Source: CAD feature listing. Evaluate the final solid. Frame: model axes, mm. A direction names the side the tool comes from. Give positions to 0.01 mm unless a question says otherwise; leave off trailing zeros. Loops run counter-clockwise (first coordinate to the right, second up) from the corner with the lowest first, then second, coordinate; pieces in that order, holes last. Notation, with made-up numbers: (43.5, -32) -> (89.5, -32) arc R24 cw to (89.5, -12) -> close; hole circle Ø10 at (28, 80.25). An arc over 180 degrees is marked (long way). Return JSON: item names as keys, results as strings. Group by question number.
(1) Cut plane A-A on z = 18.5. Return loops of the section in (x, y).
(2) Cut plane C-C on x = 22. Return loops of the section in (y, z), then the cut area to 3 significant figures.
(3) Ray query, line 1 (X direction, y = 58, z = 26); line 2 (Z direction, x = 38, y = 26.5); line 3 (Y direction, x = 54, z = 23.5). Return the intervals inside material, ascending. Write a range as from..to.
(4) Access query for faces 1 (the face through (50, 42, 12.7)), 2 (the face through (0, 38, 26)). Directions: +Z, -Z, +X, -X, +Y, -Y. A direction counts if a zero-diameter tool reaches every point of the face in a straight line with its end or side. Return the directions, or none.
(5) Cut plane B-B on y = 33. Return loops of the section in (x, z).
(6) Cut plane D-D on z = 4.5. Return loops of the section in (x, y), then the cut area to 3 significant figures.
(7) Pin query (flat end, axial travel): pin 1 (15 mm diameter, centred on x = 48, y = 40.5, fed in from +Z); pin 2 (2 mm diameter, centred on y = 50, z = 15, fed in from +X); pin 3 (3 mm diameter, centred on x = 39.5, z = 31.5, fed in from -Y). Return the tip coordinate at first contact, or that it passes through.
```python
from build123d import *

# Parameters (mm, degrees)
F0_W     = 76.2
F0_H     = 50.8
F1_DEPTH = 76.2
F2_W     = 50.8
F2_H     = 63.5
F3_DEPTH = 38.1
F5_DEPTH = 50.801


with BuildPart() as f1:
    # F0 (on Right) → F1 (new body)
    with BuildSketch(Plane.YZ):
        with Locations((38.1, 25.4)):
            Rectangle(F0_W, F0_H)
    extrude(amount=F1_DEPTH)

    # F2 (on face) → F3 (cut)
    with BuildSketch(Plane.XY.offset(50.8)):
        with Locations((50.8, 31.75)):
            Rectangle(F2_W, F2_H)
    extrude(amount=-F3_DEPTH, mode=Mode.SUBTRACT)

    # F4 (on face) → F5 (cut, through all)
    with BuildSketch(Plane.XY.offset(50.8)):
        Polygon((76.2, 25.4), (0, 0), (76.2, 0), align=None)
        Polygon((25.4, 8.466667), (25.4, 0), (76.2, 0), (76.2, 25.4), align=None)
    extrude(amount=-F5_DEPTH, mode=Mode.SUBTRACT)


solid = f1.part
```
Answers:
{
 "1": {"outline": "(0, 0) -> (25.4, 8.47) -> (25.4, 63.5) -> (76.2, 63.5) -> (76.2, 76.2) -> (0, 76.2) -> close"},
 "2": {"outline": "(7.33, 0) -> (76.2, 0) -> (76.2, 50.8) -> (7.33, 50.8) -> close", "area": "3,500 mm²"},
 "3": {"line 1": "0..25.4", "line 2": "0..12.7", "line 3": "63.5..76.2"},
 "4": {"face 1": "+Z, +X, -Y", "face 2": "+Z, -Z, -X, +Y, -Y"},
 "5": {"outline": "(0, 0) -> (76.2, 0) -> (76.2, 12.7) -> (25.4, 12.7) -> (25.4, 50.8) -> (0, 50.8) -> close"},
 "6": {"outline": "(0, 0) -> (76.2, 25.4) -> (76.2, 76.2) -> (0, 76.2) -> close", "area": "4,840 mm²"},
 "7": {"pin 1": "z = 12.7", "pin 2": "x = 25.4", "pin 3": "y = 63.5"}
}
